Build history of the part. All positions in model axes, mm. A direction names the side the tool comes from. Give positions to 0.01 mm unless a question says otherwise; leave off trailing zeros. Use a Markdown table: item, result.
from build123d import *

# Parameters (mm, degrees)
SKETCH1_W           = 5
SKETCH1_H           = 6.6
BOSS_EXTRUDE1_REACH = 70.079
SKETCH3_R           = 5
BOSS_EXTRUDE2_REACH = 83.814
SKETCH4_R           = 5
CUT_EXTRUDE1_DEPTH  = 6.6
CUT_EXTRUDE2_DEPTH  = 6.6
CUT_EXTRUDE3_DEPTH  = 6.6
CHAMFER1_SIZE       = 0.5


with BuildPart() as part:
    # Sketch1 → Revolve-Thin2 (revolve)
    with BuildSketch(Plane(origin=(0, 0, 0), x_dir=(1, 0, 0), z_dir=(0, 1, 0))):
        with Locations((-2.5, 20.8)):
            Rectangle(SKETCH1_W, SKETCH1_H)
    revolve(axis=Axis((0, 0, -17.5), (0, 0, -1)))

    # Sketch3 → Boss-Extrude1 (add, up to next)
    with BuildSketch(Plane(origin=(-38.328954944, 0, -71.518501264), x_dir=(0.881400586, 0, -0.472369565), z_dir=(0.472369565, 0, 0.881400586)), mode=Mode.PRIVATE) as boss_extrude1_sk1:
        with Locations((9.825286961, 0)):
            Circle(SKETCH3_R)
    boss_extrude1_tool1 = extrude(boss_extrude1_sk1.sketch, amount=BOSS_EXTRUDE1_REACH, mode=Mode.PRIVATE) - part.part
    add(boss_extrude1_tool1.solids().sort_by_distance((-29.668941, 0, -76.159668))[0])

    # Sketch4 → Boss-Extrude2 (add, up to next)
    with BuildSketch(Plane(origin=(38.328954944, 0, -71.518501264), x_dir=(0.881400586, 0, 0.472369565), z_dir=(-0.472369565, 0, 0.881400586)), mode=Mode.PRIVATE) as boss_extrude2_sk1:
        with Locations((-9.825286961, 0)):
            Circle(SKETCH4_R)
    boss_extrude2_tool1 = extrude(boss_extrude2_sk1.sketch, amount=BOSS_EXTRUDE2_REACH, mode=Mode.PRIVATE) - part.part
    add(boss_extrude2_tool1.solids().sort_by_distance((29.668941, 0, -76.159668))[0])

    # Sketch5 → Cut-Extrude1 (cut)
    with BuildSketch(Plane.XY.offset(-17.5)):
        Polygon((1.610807251, 2.79), (-1.610807251, 2.79), (-3.221614502, 0), (-1.610807251, -2.79), (1.610807251, -2.79), (3.221614502, 0), align=None)
    extrude(amount=-CUT_EXTRUDE1_DEPTH, mode=Mode.SUBTRACT)

    # Sketch7 → Cut-Extrude2 (cut)
    with BuildSketch(Plane(origin=(-38.328954944, 0, -71.518501264), x_dir=(-0.881400586, 0, 0.472369565), z_dir=(-0.472369565, 0, -0.881400586))):
        Polygon((-7.035286961, 1.610807251), (-9.825286961, 3.221614502), (-12.615286961, 1.610807251), (-12.615286961, -1.610807251), (-9.825286961, -3.221614502), (-7.035286961, -1.610807251), align=None)
    extrude(amount=-CUT_EXTRUDE2_DEPTH, mode=Mode.SUBTRACT)

    # Sketch8 → Cut-Extrude3 (cut)
    with BuildSketch(Plane(origin=(38.328954944, 0, -71.518501264), x_dir=(-0.881400586, 0, -0.472369565), z_dir=(0.472369565, 0, -0.881400586))):
        Polygon((12.615286961, 1.610807251), (9.825286961, 3.221614502), (7.035286961, 1.610807251), (7.035286961, -1.610807251), (9.825286961, -3.221614502), (12.615286961, -1.610807251), align=None)
    extrude(amount=-CUT_EXTRUDE3_DEPTH, mode=Mode.SUBTRACT)

    # Chamfer1
    chamfer1_edges = [part.edges().sort_by_distance(p)[0] for p in [
        (2.416210877, 1.395, -17.5),
        (0, 2.79, -17.5),
        (-2.416210877, 1.395, -17.5),
        (-2.416210877, -1.395, -17.5),
        (0, -2.79, -17.5),
        (2.416210877, -1.395, -17.5),
        (-32.128048891, 0, -74.841756709),
        (-30.898495073, 2.416210877, -75.500712253),
        (-28.439387437, 2.416210877, -76.81862334),
        (-27.209833619, 0, -77.477578884),
        (-28.439387437, -2.416210877, -76.81862334),
        (-30.898495073, -2.416210877, -75.500712253),
        (27.209833619, 0, -77.477578884),
        (28.439387437, 2.416210877, -76.81862334),
        (30.898495073, 2.416210877, -75.500712253),
        (32.128048891, 0, -74.841756709),
        (30.898495073, -2.416210877, -75.500712253),
        (28.439387437, -2.416210877, -76.81862334),
    ]]
    chamfer(chamfer1_edges, length=CHAMFER1_SIZE)


solid = part.part
1) Pin check, flat tips, straight feed: P1, Ø6, axis at x = 8, y = -3, coming from the -Z side; P2, Ø3, axis at y = -1, z = -41.5, coming from the -X side; P3, Ø3, axis at y = 1.5, z = -33, coming from the +X side. Stop position of each tip, or through.
Computed:
| item | result |
|---|---|
| P1 | stops at z = -50.73 |
| P2 | stops at x = -17.5 |
| P3 | stops at x = 12.86 |
2) Wall check: line 1 (X direction, y = -1.5, z = -70.5); line 2 (X direction, y = 2.25, z = -44.5); line 3 (X direction, y = 1.5, z = -49.5). Give the ranges that are in metal, low to high. Write a range as from..to.
Computed:
| item | result |
|---|---|
| line 1 | x = -32.05..-29.8, -26.26..-21.22, 21.22..26.26, 29.8..32.05 |
| line 2 | x = -17.77..-7.64, 7.64..17.77 |
| line 3 | x = -20.79..-9.97, 9.97..20.79 |
3) Tool access for faces 1 (the flat face through (-30.5, 0, -71.8)), 2 (the flat face through (2.405, -1.415, -21.007)), 3 (the flat face through (-26.8, 2.427, -73.718)): list every direction of +Z, -Z, +X, -X, +Y, -Y with a clear straight run to the whole face (end or side of a thin tool).
Computed:
| item | result |
|---|---|
| face 1 | -Z |
| face 2 | +Z |
| face 3 | none |
4) Two-plate mould, pull along Y, no slides. Class faces 4 (the cylindrical face through (0, 5, -23)), 5 (the flat face through (-28.23, 2.64, -76.64)), 6 (the cylindrical face through (0, -5, -23)): +Y half, -Y half, draft (parallel to the pull), parting line (faces both ways), or undercut.
Computed:
| item | result |
|---|---|
| face 4 | +Y half |
| face 5 | undercut |
| face 6 | -Y half |
